Autodesk Inventor part; units mm, degrees
ref_plane "YZ Plane" through (0, 0, 0) normal (1, 0, 0) x (0, 1, 0)
ref_plane "XZ Plane" through (0, 0, 0) normal (0, 1, 0) x (-1, 0, 0)
ref_plane "XY Plane" through (0, 0, 0) normal (0, 0, 1) x (1, 0, 0)
sketch "Náčrt1" plane through (0, 0, 0) normal (0, 1, 0) x (-1, 0, 0)
  line L0 (0, 0) -> (49.75, 0)
  line L1 (49.75, 0) -> (49.75, -40)
  line L2 (49.75, -40) -> (0, -40)
  line L3 (0, -1) -> (49.75, -1)
  line L4 (18, -36) -> (16, -36)
  line L5 (18, -36) -> (18, -39.9)
  line L6 (18, -39.9) -> (16, -39.9)
  line L7 (16, -39.9) -> (16, -36)
  line L8 (5.25, -40) -> (5.25, -36)
  line L9 (5.25, -36) -> (9.75, -36)
  line L10 (9.75, -36) -> (9.75, -40)
  line L11 (0, -4) -> (26, -4)
  line L12 (26, -4) -> (26, -31)
  line L13 (26, -31) -> (0, -31)
  line L14 (0, -40) -> (0, -31)
  line L15 (0, -4) -> (0, 0)
  line L16 (33, -13.5) -> (31, -13.5)
  line L17 (31, -13.5) -> (31, -21.5)
  line L18 (31, -21.5) -> (33, -21.5)
  line L19 (33, -21.5) -> (33, -13.5)
  point P0 (49.75, -20)
  point P1 (33, -17.5)
  point P2 (26, -17.5)
  dimension "d0" = 40
  dimension "d1" = 49.75
  dimension "d2" = 1
  dimension "d5" = 4
  dimension "d16" = 0.1
  dimension "d17" = 31.75
  dimension "d18" = 2
  dimension "d28" = 4.5
  dimension "d29" = 4
  dimension "d57" = 27
  dimension "d58" = 26
  dimension "d59" = 5.25
  dimension "d60" = 8
  dimension "d61" = 2
  dimension "d62" = 5
  dimension "d63" = 4
extrude "Vysunutí1" add sketch "Náčrt1" along normal blind 2.5 contours L3 L1 L2 L10 L9 L8 L14 L13 L12 L11 L15 | L2 L8 L9 L10 | L5 L6 L7 L4
extrude "Vysunutí2" add sketch "Náčrt1" along normal blind 1.25 contours L0 L1 L3 L15
extrude "Vysunutí3" add sketch "Náčrt1" against normal blind 12.5 contours L5 L6 L7 L4
sketch "Náčrt3" plane through (-16, 0, -39.9) normal (0, 0, -1) x (-1, 0, 0)
  line L0 (0, 0) -> (0, -12.5)
  line L1 (0, -12.5) -> (2, -12.5)
  line L2 (2, 0) -> (2, -12.5)
  line L3 (0, 0) -> (0, -12.5)
  line L4 (0, -10.6) -> (2, -10.6)
  line L5 (2, 0) -> (2, -12.5)
  point P0 (-16, 0)
  point P1 (2, -10.6)
  point P2 (0, -10.6)
  dimension "d19" = 1.9
extrude "Vysunutí5" add sketch "Náčrt3" along normal blind 5
fillet "Zaoblení1" radius 1 1 edges at (-49.75, 1.25, -40)
extrude "Vysunutí6" add sketch "Náčrt1" against normal blind 8 contours L2 L8 L9 L10
sketch "Náčrt7" plane through (-5.25, -8, -36) normal (1, 0, 0) x (0, 0, -1)
  line L0 (0, 8) -> (0, 0)
  line L1 (0, 0) -> (4, 0)
  line L2 (4, 8) -> (4, 0)
  line L3 (0, 8) -> (0, 0)
  line L4 (0, 2) -> (4, 2)
  line L5 (4, 8) -> (4, 0)
  point P0 (-36, 8)
  dimension "d36" = 2
extrude "Vysunutí8" add sketch "Náčrt7" along normal up to surface (5.25 mm away)
sketch "Náčrt8" plane through (0, 0, -40) normal (0, 0, -1) x (-1, 0, 0)
  line L0 (9.75, 0) -> (9.75, -8)
  line L1 (5.25, -6) -> (0, -6)
  point P0 (0, 0)
  point P1 (7.5, -3)
  dimension "d46" = 2.25
  dimension "d47" = 3
hole "Díra1" at (-7.5, -3, -40) direction (0, 0, 1) diameter 2 end through all
mirror "Zrcadlit2" about plane through (0, 0, -40) normal (1, 0, 0)
properties part number "Kryt těla"
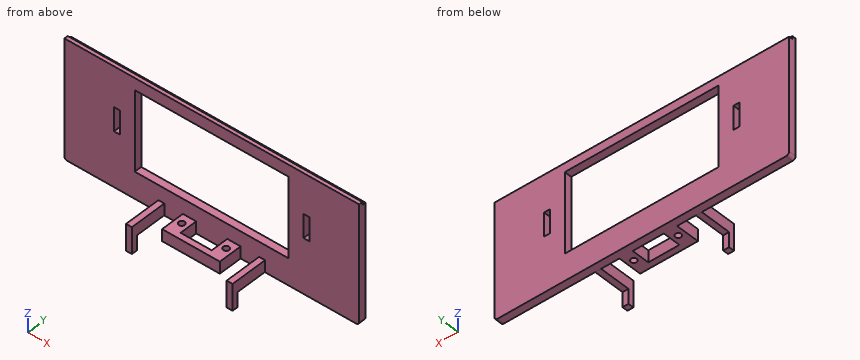
The listing builds one solid part. Answer for the finished solid, in the listing's coordinates (mm). Give positions to 0.01 mm unless a question says otherwise; leave off trailing zeros. Order: outer loops, then holes, each group sorted by start corner. A loop starts at its lowest first (then second) coordinate and runs counter-clockwise, first axis right, second up. Notation, with made-up numbers: (75.25, 50.25) - (82.25, 50.25) arc R25 cw to (82.25, 63.25) - close; hole circle Ø6 at (-9, 39). An arc over 180 degrees is marked (long way). Use one line per item in the form item = value.
1) Find section D-D on x = -13.5. Determine the outline of the cut face in (y, z).
Verdict:
outline = (0, -40) - (2.5, -40) - (2.5, -31) - (0, -31) - close; (0, -4) - (2.5, -4) - (2.5, -1) - (1.25, -1) - (1.25, 0) - (0, 0) - close
2) Find section A-A on y = -3. Determine the outline of the cut face in (x, z), and give its area (3 significant figures).
Verdict:
outline = (-18, -39.9) - (-16, -39.9) - (-16, -36) - (-18, -36) - close; (-9.75, -40) - (-8.5, -40) - (-8.5, -36) - (-9.75, -36) - close; (-6.5, -40) - (-5.25, -40) - (-5.25, -36) - (-6.5, -36) - close; (5.25, -40) - (6.5, -40) - (6.5, -36) - (5.25, -36) - close; (8.5, -40) - (9.75, -40) - (9.75, -36) - (8.5, -36) - close; (16, -39.9) - (18, -39.9) - (18, -36) - (16, -36) - close
area = 35.6 mm^2
3) Consider probe 1 along X at (y, z) = (-3, -38.45); probe 2 along Z at (x, y) = (-15, 1.5); probe 3 along Z at (x, y) = (-32, 2.25). Determine where each line is inside the solid, lowest interval first. Write a range as [from, to].
Verdict:
probe_1 = [-18, -16], [-9.75, -8.5], [-6.5, -5.25], [5.25, 6.5], [8.5, 9.75], [16, 18]
probe_2 = [-40, -31], [-4, -1]
probe_3 = [-40, -21.5], [-13.5, -1]
4) Find section B-B on z = -6. Determine the outline of the cut face in (x, y).
Verdict:
outline = (-49.75, 0) - (-26, 0) - (-26, 2.5) - (-49.75, 2.5) - close; (26, 0) - (49.75, 0) - (49.75, 2.5) - (26, 2.5) - close
5) Find section C-C on x = 7.5. Determine the outline of the cut face in (y, z), and give its area (4 significant figures).
Verdict:
outline = (-8, -40) - (-4, -40) - (-4, -36) - (-8, -36) - close; (-2, -40) - (2.5, -40) - (2.5, -31) - (0, -31) - (0, -36) - (-2, -36) - close; (0, -4) - (2.5, -4) - (2.5, -1) - (1.25, -1) - (1.25, 0) - (0, 0) - close
area = 55.25 mm^2
6) Each of these flat-tipped pins is pushed along its axis until it touches: pin 1 (3 mm diameter, centred on y = -2.5, z = -38, fed in from +X); pin 2 (7 mm diameter, centred on y = -3.5, z = -41, fed in from -X); pin 3 (4 mm diameter, centred on x = -4, z = -30.5, fed in from -Y). Where does it stop, or does it pass through?
Verdict:
pin_1 = 18
pin_2 = -18
pin_3 = 0
